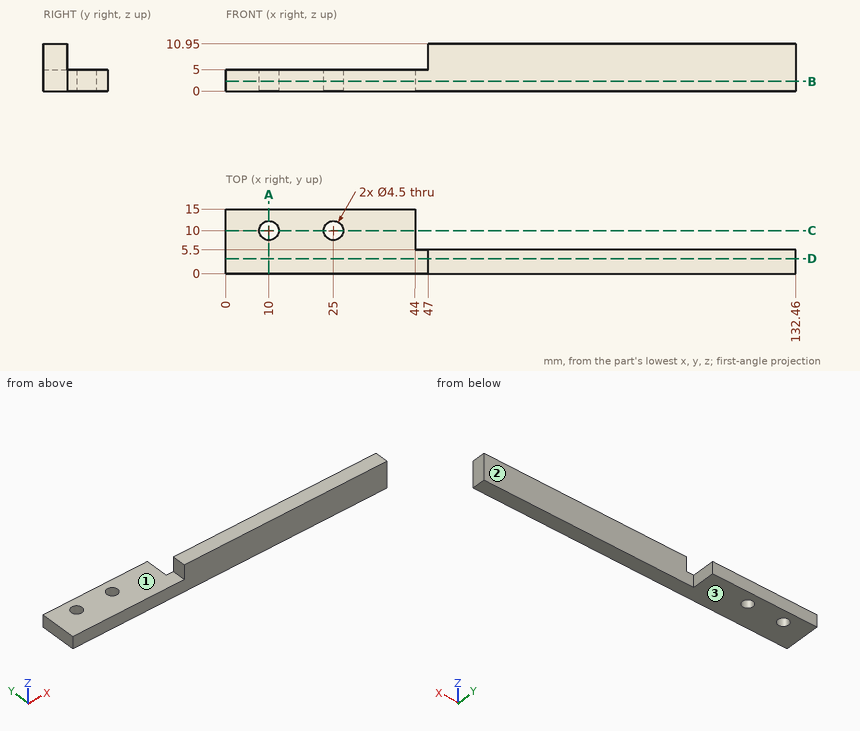
Drawing for the job (mm, zero at the part's lowest x, y, z). A direction names the side the tool comes from. Give positions to 0.01 mm unless a question says otherwise; leave off trailing zeros. Write each loop counter-clockwise with the first axis right and the second up, starting at its lowest first coordinate (ties: lowest second). Pieces come first, ordered by that corner, then holes. Notation, with made-up numbers: M -23,17.25 L -13,17.25 A19 ccw -13,30.25 Z; hole C -3.5,89 d1. An arc over 180 degrees is marked long. Return JSON: item names as keys, results as strings. Group by question number.
(1) Drill centre lines: L1, parallel to Y at x = 25, z = 1.5; L2, parallel to X at y = 9.5, z = 4.5; L3, parallel to Y at x = 90, z = 9.75. Where is each one in solid material? Low to high. Write a range as [from, to].
(2) Band-saw the part on B-B (z = 2.25). Give the cut face in (x, y), and give its area (3 significant figures).
(3) Flat gauge pins, fed straight in: pin 1 Ø3 at (y, z) = (3, 7) entering from -X; pin 2 Ø7.5 at (x, y) = (19, 11) entering from +Z; pin 3 Ø1.5 at (y, z) = (8, 1.5) entering from +X; pin 4 Ø6 at (x, y) = (117, 8) entering from +Z. Where does each tip first touch, or does it go through?
(4) Band-saw the part on D-D (y = 3.5). Give the cut face in (x, z).
(5) Band-saw the part on A-A (x = 10). Give the cut face in (y, z), and give its area (3 significant figures).
(6) Band-saw the part on C-C (y = 10). Give the cut face in (x, z), and give its area (3 significant figures).
(7) 3-axis set-ups, long thin cutter, end or side, ignore diameter. For the marked faces 1, 2 and 3: which of +Z, -Z, +X, -X, +Y, -Y reach the whole face in a straight line?
Entries:
{
 "1": {"L1": "y = [0, 7.75], [12.25, 15]", "L2": "x = [0, 7.81], [12.19, 22.81], [27.19, 44]", "L3": "y = [0, 5.5]"},
 "2": {"outline": "M 0,0 L 132.46,0 L 132.46,5.5 L 44,5.5 L 44,15 L 0,15 Z; hole C 10,10 d4.5; hole C 25,10 d4.5", "area": "1,110 mm^2"},
 "3": {"pin 1": "stops at x = 47", "pin 2": "stops at z = 5", "pin 3": "stops at x = 44", "pin 4": "stops at z = 10.95"},
 "4": {"outline": "M 0,0 L 132.46,0 L 132.46,10.95 L 47,10.95 L 47,5 L 0,5 Z"},
 "5": {"outline": "M 0,0 L 7.75,0 L 7.75,5 L 0,5 Z; M 12.25,0 L 15,0 L 15,5 L 12.25,5 Z", "area": "52.5 mm^2"},
 "6": {"outline": "M 0,0 L 7.75,0 L 7.75,5 L 0,5 Z; M 12.25,0 L 22.75,0 L 22.75,5 L 12.25,5 Z; M 27.25,0 L 44,0 L 44,5 L 27.25,5 Z", "area": "175 mm^2"},
 "7": {"face 1": "+Z, -X, +Y, -Y", "face 2": "+Z, -Z, +X, +Y", "face 3": "-Z, +X, -X, +Y, -Y"}
}
